Verification items for the finished model (mm, model axes). Face numbers are marked on the shaded views. Give positions to 0.01 mm unless a question says otherwise; leave off trailing zeros. Use one line per item in the form item = value.
```python
from build123d import *

# Parameters (mm, degrees)
F1_DEPTH = 6.35
F3_D     = 11.43
F3_DEPTH = 25.4


with BuildPart() as f1:
    # F0 (on Front) → F1 (new body)
    with BuildSketch(Plane.XZ):
        with BuildLine():
            ThreePointArc((-35.819092, 15.691353), (-34.365454, 17.786657), (-33.853378, 20.284886))
            ThreePointArc((-33.853378, 20.284886), (-34.365454, 22.783114), (-35.819092, 24.878418))
            ThreePointArc((-35.819092, 24.878418), (-40.203378, 26.634886), (-44.587663, 24.878418))
            ThreePointArc((-44.587663, 24.878418), (-46.548686, 20.528945), (-44.927549, 16.041691))
            add(Edge.make_bspline(
                [(-44.927549, 16.041691), (-44.81393, 15.92811), (-44.700614, 15.81136), (-44.587663, 15.691353)],
                knots=[25.075757, 25.075757, 25.075757, 25.075757, 25.337787, 25.337787, 25.337787, 25.337787], degree=3))
            ThreePointArc((-44.587663, 15.691353), (-40.203378, 13.934886), (-35.819092, 15.691353))
        make_face()
        with BuildLine():
            ThreePointArc((-44.587663, 24.878418), (-40.203378, 26.634886), (-35.819092, 24.878418))
            add(Edge.make_bspline(
                [(-44.587663, 24.878418), (-38.347919, 30.843824), (-43.083301, 42.885957), (-36.29899, 31.356057), (-35.819092, 24.878418)],
                knots=[0, 0, 0, 0, 12.88347, 25.76694, 25.76694, 25.76694, 25.76694], degree=3))
        make_face()
        with BuildLine():
            ThreePointArc((-44.927549, 16.041691), (-46.548686, 20.528945), (-44.587663, 24.878418))
            add(Edge.make_bspline(
                [(-44.587663, 24.878418), (-50.169606, 23.91101), (-62.550365, 17.929967), (-50.307292, 21.41963), (-44.927549, 16.041691)],
                knots=[0, 0, 0, 0, 12.668893, 25.075757, 25.075757, 25.075757, 25.075757], degree=3))
        make_face()
        with BuildLine():
            add(Edge.make_bspline(
                [(-44.587663, 15.691353), (-43.733824, 9.608083), (-37.574358, -1.828031), (-41.93097, 9.608083), (-35.819092, 15.691353)],
                knots=[0, 0, 0, 0, 12.589411, 25.178822, 25.178822, 25.178822, 25.178822], degree=3))
            ThreePointArc((-35.819092, 15.691353), (-40.203378, 13.934886), (-44.587663, 15.691353))
        make_face()
        with BuildLine():
            ThreePointArc((-35.819092, 24.878418), (-34.365454, 22.783114), (-33.853378, 20.284886))
            ThreePointArc((-33.853378, 20.284886), (-34.365454, 17.786657), (-35.819092, 15.691353))
            add(Edge.make_bspline(
                [(-35.819092, 24.878418), (-28.212329, 18.476849), (-17.657736, 22.999454), (-28.212329, 16.663786), (-35.819092, 15.691353)],
                knots=[0, 0, 0, 0, 13.678433, 27.356866, 27.356866, 27.356866, 27.356866], degree=3))
        make_face()
    extrude(amount=F1_DEPTH)

    # F3
    with Locations(Plane.XZ.offset(6.35)):
        with Locations((-40.305141, 20.274019)):
            Hole(F3_D / 2, depth=F3_DEPTH)


solid = f1.part
```
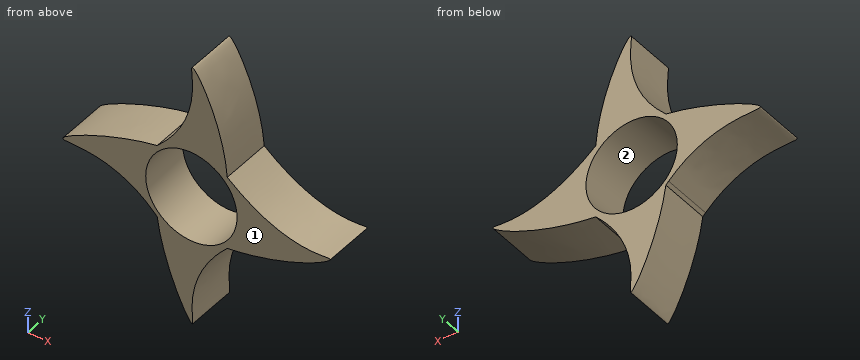
1. Depth check by flat-ended pin: pin 1 Ø2 at (x, y) = (-33.5, -2.5) entering from +Z; pin 2 Ø1 at (y, z) = (-4.5, 7.5) entering from +X. Enter the tip coordinate at first touch or a pass-through.
Result set:
pin_1 = 23.84
pin_2 = -40.06
2. Scan lines: probe 1 along Z at (x, y) = (-42, -4.5); probe 2 along Z at (x, y) = (-41.5, -0.5); probe 3 along Z at (x, y) = (-50.5, -6). Record each from-to range of solid material in increasing order.
Result set:
probe_1 = 6.95 to 14.82, 25.73 to 28.05
probe_2 = 5.89 to 14.69, 25.86 to 28.95
probe_3 = 19.47 to 23.26
3. Draft check along X on the marked faces 1 and 2. Enter one of: released by +X, released by -X, zero draft, split by the parting line, or undercut.
Result set:
face_1 = zero draft
face_2 = undercut
